The listing builds one solid part. Answer for the finished solid, in the listing's coordinates (mm). Face numbers are marked on the shaded views. A direction names the side the tool comes from. Coordinates: 2 decimals unless noted, no trailing zeros. Order: outer loops, then holes, each group sorted by start corner. A loop starts at its lowest first (then second) coordinate and runs counter-clockwise, first axis right, second up. Notation, with made-up numbers: (-28.75, 41.25) -> (-10.75, 41.25) arc R18 cw to (-10.75, 62.25) -> close; hole circle Ø8 at (-4.5, 57.25). An arc over 180 degrees is marked (long way). Return JSON: item names as keys, results as strings.
```python
from build123d import *

# Parameters (mm, degrees)
F0_W     = 76.2637332082
F0_H     = 33.6211510003
F0_W_2   = 76.2320831418
F0_H_2   = 42.8359024227
F1_DEPTH = 25.4
F2_R     = 12.7


with BuildPart() as f1:
    # F0 (on Front) → F1 (new body)
    with BuildSketch(Plane.XZ):
        with BuildLine():
            Line((-76.2637332082, 33.6211510003), (0, 33.6211510003))
            Line((0, 33.6211510003), (0, 76.4570534229))
            ThreePointArc((0, 76.4570534229), (-43.7352018951, 65.015109335), (-76.2637332082, 33.6211510003))
        make_face()
        with Locations((-38.1318666041, 16.8105755001)):
            Rectangle(F0_W, F0_H)
        with Locations((38.1160415709, 16.8105755001)):
            Rectangle(F0_W_2, F0_H)
        with Locations((38.1160415709, 55.0391022116)):
            Rectangle(F0_W_2, F0_H_2)
        Polygon((76.2320831418, 33.6211510003), (76.2320831418, 0), (153.9078503847, 0), (153.9078503847, 33.6211510003), (115.0699667633, 33.6211510003), align=None)
        with BuildLine():
            Line((76.2320831418, 76.4570534229), (76.2320831418, 33.6211510003))
            Line((76.2320831418, 33.6211510003), (115.0699667633, 33.6211510003))
            ThreePointArc((115.0699667633, 33.6211510003), (87.3870520199, 47.5464336589), (76.2320831418, 76.4570534229))
        make_face()
    extrude(amount=F1_DEPTH)

    # F2
    f2_edges = [f1.edges().sort_by_distance(p)[0] for p in [
        (153.90785, -12.7, 33.621151),
    ]]
    fillet(f2_edges, radius=F2_R)


solid = f1.part
```
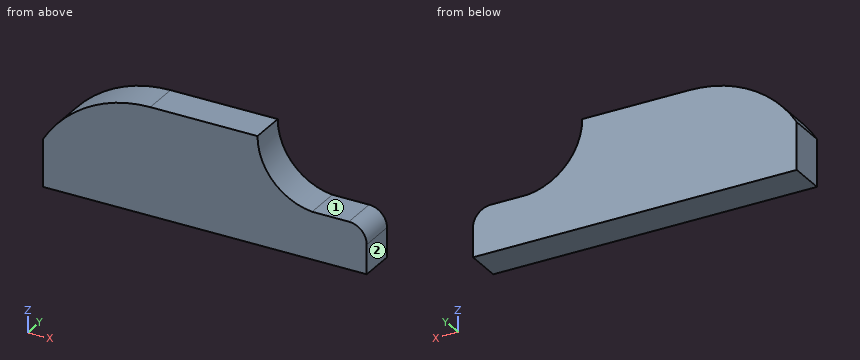
Item 1: Flat-ended cylindrical pins translate along their axes: pin 1 (4 mm diameter, centred on x = 97.5, y = -8, fed in from +Z); pin 2 (3 mm diameter, centred on y = -18.5, z = 51.5, fed in from -X). Find the tip coordinate at first contact, or state that the pin passes through.
Answer list:
{"pin 1": "z = 40.58", "pin 2": "x = -63.45"}
Item 2: The part is cut by section B-B on x = 117.5. Determine the outline of the cut face in (y, z).
Answer list:
{"outline": "(-25.4, 0) -> (0, 0) -> (0, 33.62) -> (-25.4, 33.62) -> close"}
Item 3: Which of the six approach directions +Z, -Z, +X, -X, +Y, -Y give full straight-line access (tool end or side, diameter ignored) to the marked faces 1 and 2?
Answer list:
{"face 1": "+Z, +X, +Y, -Y", "face 2": "+Z, -Z, +X, +Y, -Y"}
Item 4: The part is cut by section A-A on y = -5.5. Determine the outline of the cut face in (x, z), plus the area to 3 significant figures.
Answer list:
{"outline": "(-76.26, 0) -> (153.91, 0) -> (153.91, 20.92) arc R12.7 ccw to (141.21, 33.62) -> (115.07, 33.62) arc R43.04 cw to (76.23, 76.46) -> (0, 76.46) arc R89.31 ccw to (-76.26, 33.62) -> close", "area": "13,700 mm2"}
Item 5: Find the intervals of material crossed by probe 1 along Z at (x, y) = (138.5, -19); probe 2 along Z at (x, y) = (-50.5, -15.5); probe 3 along X at (y, z) = (-11.5, 68), in increasing order.
Answer list:
{"probe 1": "0 to 33.62", "probe 2": "0 to 60.81", "probe 3": "-37.93 to 77.07"}
Item 6: The part is cut by section C-C on z = 30.5. Determine the outline of the cut face in (x, y), plus the area to 3 significant figures.
Answer list:
{"outline": "(-76.26, -25.4) -> (149.55, -25.4) -> (149.55, 0) -> (-76.26, 0) -> close", "area": "5,740 mm2"}
